Source: three-view drawing plus pictorial views. Frame: mm from the lowest corner of the part. A direction names the side the tool comes from. Round coordinates to 2 decimals unless told otherwise and drop trailing zeros. Loops run counter-clockwise (first coordinate to the right, second up) from the corner with the lowest first, then second, coordinate; pieces in that order, holes last. Notation, with made-up numbers: (-38, 61) -> (-19, 61) arc R28 ccw to (-19, 98) -> close; hole circle Ø8 at (31.25, 85.5). An arc over 180 degrees is marked (long way). One line per question, with ' | ' between items. Start each with the question number.
Q1. Material intervals for L1, parallel to Z at x = 250, y = 11.5; L2, parallel to Y at x = 213.5, z = 250, sorted ascending.
Q2. Cut plane C-C on z = 302. Return loops of the section in (x, y), and give its area (3 significant figures).
Q3. Cut plane B-B on z = 188.5. Return loops of the section in (x, y).
Q4. Mould query, pull axis X, two halves, no side actions, for the marked faces 1, 2, 3 and 4. Classes: pulls with the +X half, pulls with the -X half, needs draft (parallel to the pull), parting line crosses it, or undercut.
Q5. Contact query for flat-ended pins moving along their axis: P1, Ø3, axis at x = 160.5, z = 102.5, coming from the -Y side; P2, Ø5, axis at x = 313.5, z = 348, coming from the -Y side; P3, Ø1, axis at x = 201.5, y = 424.5, coming from the -Z side; P4, Ø1.5, axis at x = 251, y = 125, coming from the -Z side. Output: stop coordinate, or through.
Q6. Access query for the marked faces 5, 6 and 7. Directions: +Z, -Z, +X, -X, +Y, -Y. A direction counts if a zero-diameter tool reaches every point of the face in a straight line with its end or side. Return the directions, or none.
Q7. Cut plane D-D on x = 410.5. Return loops of the section in (y, z).
Q8. Cut plane A-A on y = 405. Return loops of the section in (x, z).
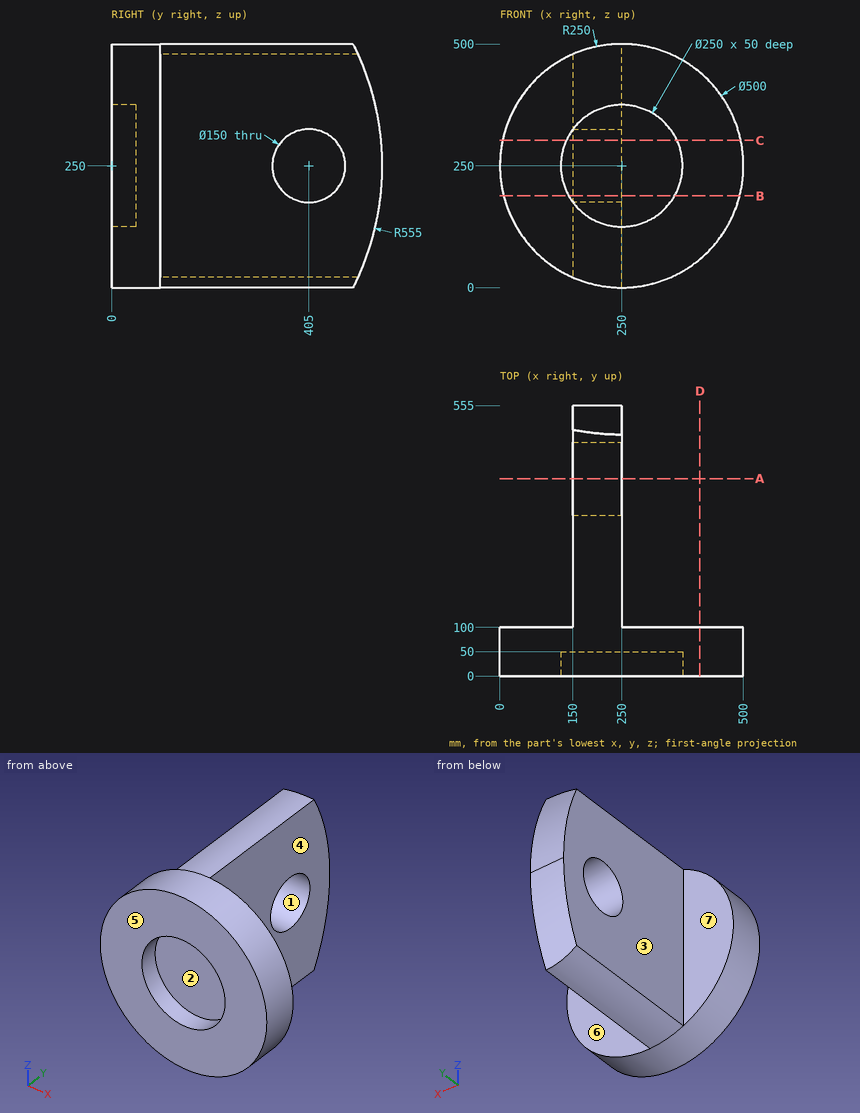
Results:
1) L1: 0 to 125, 375 to 500 | L2: 50 to 330, 480 to 555
2) outline: (5.47, 0) -> (136.33, 0) -> (136.33, 50) -> (363.67, 50) -> (363.67, 0) -> (494.53, 0) -> (494.53, 100) -> (250, 100) -> (250, 350.95) -> (150, 350.95) -> (150, 100) -> (5.47, 100) -> close; (150, 459.05) -> (250, 459.05) -> (250, 552.56) -> (150, 552.56) -> close | area: 72,000 mm^2
3) outline: (7.68, 0) -> (141.18, 0) -> (141.18, 50) -> (358.82, 50) -> (358.82, 0) -> (492.32, 0) -> (492.32, 100) -> (250, 100) -> (250, 362.07) -> (150, 362.07) -> (150, 100) -> (7.68, 100) -> close; (150, 447.93) -> (250, 447.93) -> (250, 551.58) -> (150, 551.58) -> close
4) face 1: needs draft | face 2: undercut | face 3: pulls with the -X half | face 4: pulls with the +X half
5) P1: y = 0 | P2: y = 50 | P3: z = 4.65 | P4: through
6) face 5: +Z, -Z, +X, -X, -Y | face 6: +Z, -Z, +X, +Y | face 7: +Z, -Z, -X, +Y
7) outline: (0, 58.32) -> (100, 58.32) -> (100, 441.68) -> (0, 441.68) -> close
8) outline: (150, 20.87) arc R250 ccw to (250, 0) -> (250, 175) -> (150, 175) -> close; (150, 325) -> (250, 325) -> (250, 500) arc R250 ccw to (150, 479.13) -> close
